Autodesk Inventor part; units mm, degrees
ref_plane "YZ Plane" through (0, 0, 0) normal (1, 0, 0) x (0, 1, 0)
ref_plane "XZ Plane" through (0, 0, 0) normal (0, 1, 0) x (-1, 0, 0)
ref_plane "XY Plane" through (0, 0, 0) normal (0, 0, 1) x (1, 0, 0)
sketch "Sketch1" plane through (0, 0, 0) normal (0, 0, 1) x (1, 0, 0)
  line L0 (-750, 67.5235) -> (750, 67.5235)
  line L1 (750, 67.5235) -> (750, 0)
  line L2 (750, 0) -> (-750, 0)
  line L3 (-750, 0) -> (-750, 67.5235)
  point P0 (0, 0)
  point P1 (0, 0)
  dimension "d0" = 1500
  dimension "d1" = 67.5235
extrude "Plate1" add sketch "Sketch1" along normal blind 2
sketch "Sketch2" plane through (750, 2, 0) normal (0, -1, 0) x (1, 0, 0)
  line L0 (-1500, 0) -> (0, 0)
  line L1 (0, 0) -> (0, 30)
  line L2 (0, 30) -> (-1500, 30)
  line L3 (-1500, 30) -> (-1500, 0)
edge flange "Flange1" height 30 angle 90 thickness 2 bend radius 2.75 thickness toward (0, -1, 0) relief round relief width 2 relief depth 1 edges at (0, 0, 2) wall of the first edge with corners at (-750, 2, 0) (750, 2, 0) (750, 2, 30) (-750, 2, 30)
bend "Bend1"
corner "Corner1"
sketch "Sketch5" plane through (0, 0, 0) normal (0, 0, -1) x (-1, 0, 0)
  line L0 (750, 67.5235) -> (-750, 67.5235)
  line L1 (-1, 30) -> (-1, 67.5235)
  line L2 (750, 0) -> (-750, 0)
  line L3 (-1, 30) -> (1, 30)
  line L4 (1, 30) -> (1, 67.5235)
  point P0 (0, 0)
  point P1 (0, 30)
  point P2 (0, 0)
  dimension "d27" = 2
  dimension "d28" = 30
extrude "Extrusion1" cut sketch "Sketch5" against normal through all
pattern_linear "Rectangular Pattern1" count 3 spacing 500 along (1, 0, 0) of "Extrusion1" first direction both ways yes
sketch "Sketch6" plane through (0, 0, 0) normal (0, 0, -1) x (-1, 0, 0)
  line L0 (-750, 67.5235) -> (-750, 4.75)
  circle A0 centre (-750, 67.5235) radius 22.5
  line L1 (-750, 67.5235) -> (750, 67.5235)
  line L2 (-1, 30) -> (-1, 67.5235)
  line L3 (-499, 67.5235) -> (-499, 30)
  line L4 (-1, 30) -> (-499, 30) construction
  circle A1 centre (-250, 67.5235) radius 22.5
  point P0 (0, 0)
  point P1 (-727.5, 67.5235)
  point P2 (-750, 45.0235)
  point P3 (-250, 30)
  dimension "d24" = 45
extrude "Extrusion2" cut sketch "Sketch6" along normal mid plane 30 contours L1 A0 L0 | A1 L1 | L1 A1 picked at (-748.3311, 52.7115)
mirror "Mirror1" about plane through (0, 0, 0) normal (1, 0, 0) of "Extrusion2"
sketch "Sketch7" plane through (0, 0, 2) normal (0, 0, 1) x (1, 0, 0)
  arc A0 (-750, 45.0235) -> (-727.5, 67.5235) centre (-750, 67.5235) ccw
  line L0 (-750, 4.75) -> (-750, 45.0235)
  line L1 (-750, 4.75) -> (750, 4.75)
  line L2 (750, 45.0235) -> (750, 4.75)
  arc A1 (727.5, 67.5235) -> (750, 45.0235) centre (750, 67.5235) ccw
  line L3 (501, 67.5235) -> (727.5, 67.5235)
  line L4 (501, 67.5235) -> (501, 30)
  line L5 (501, 30) -> (499, 30)
  line L6 (499, 30) -> (499, 67.5235)
  line L7 (1, 67.5235) -> (227.5, 67.5235)
  line L8 (1, 67.5235) -> (1, 30)
  line L9 (1, 30) -> (-1, 30)
  line L10 (-1, 30) -> (-1, 67.5235)
  line L11 (-499, 67.5235) -> (-272.5, 67.5235)
  line L12 (-499, 67.5235) -> (-499, 30)
  line L13 (-499, 30) -> (-501, 30)
  line L14 (-501, 30) -> (-501, 67.5235)
  line L15 (-727.5, 67.5235) -> (-501, 67.5235)
  line L16 (650, 4.75) -> (650, 67.5235) construction
  line L17 (-750, 4.75) -> (750, 4.75)
  circle A2 centre (650, 36.1368) radius 5
  line L18 (272.5, 67.5235) -> (499, 67.5235)
  arc A3 (227.5, 67.5235) -> (272.5, 67.5235) centre (250, 67.5235) ccw
  line L19 (-227.5, 67.5235) -> (-1, 67.5235)
  arc A4 (-272.5, 67.5235) -> (-227.5, 67.5235) centre (-250, 67.5235) ccw
  point P0 (0, 0)
  dimension "d29" = 100
  dimension "d30" = 10
extrude "Extrusion3" [suppressed]
mirror "Mirror2" [suppressed]
sketch "Sketch8" plane through (0, 0, 2) normal (0, 0, 1) x (1, 0, 0)
  line L0 (494, 62.5235) -> (494, 50.5235) construction
  line L1 (494, 50.5235) -> (294, 50.5235) construction
  line L2 (294, 50.5235) -> (294, 62.5235) construction
  line L3 (294, 62.5235) -> (494, 62.5235) construction
  line L4 (501, 67.5235) -> (727.5, 67.5235)
  line L5 (272.5, 67.5235) -> (499, 67.5235)
  point P0 (0, 0)
  dimension "d33" = 200
  dimension "d34" = 12
  dimension "d37" = 5
  dimension "d38" = 5
mark "Mark2"
equation "\"d1\" = Стрингер_3"
equation "\"d27\" = d18"
equation "\"d2\" = Thickness"
equation "\"d3\" = BendReliefWidth"
equation "\"d4\" = BendReliefDepth"
equation "\"d5\" = MinimumRemnant"
equation "\"d6\" = TransitionRadius"
equation "\"d9\" = BendRadius"
equation "\"d10\" = CornerReliefSize"
equation "\"d11\" = GapSize"
equation "\"d12\" = JacobiRadiusSize"
equation "\"BendReliefWidth\" = Thickness"
equation "\"BendReliefDepth\" = 0.5 * Thickness"
equation "\"CornerReliefSize\" = 4 * Thickness"
equation "\"MinimumRemnant\" = 2 * Thickness"
equation "\"TransitionRadius\" = BendRadius"
equation "\"JacobiRadiusSize\" = BendRadius"
equation "\"GapSize\" = Thickness"
equation "\"d18\" = Thickness"
properties part number "MSC 053 stringer board #" material "Stainless Steel"
Read the model definition and answer for the solid it produces. Units are mm, in the model's axes. A direction names the side the tool comes from. Round coordinates to 2 decimals unless told otherwise and drop trailing zeros. Order: outer loops, then holes, each group sorted by start corner. A loop starts at its lowest first (then second) coordinate and runs counter-clockwise, first axis right, second up.
1) The part is cut by section A-A on y = 55.5. Write down the section's boundary in (x, z).
2) Straight lines are drawn through the part: L1, parallel to Y at x = -579, z = 24.5; L2, parallel to Y at x = -668.5, z = 1.5. For each, find the intervals that lie inside material, in ascending order.
3) The part is cut by section B-B on x = -250. Write down the section's boundary in (y, z).
4) The part is cut by section D-D on x = -412. Write down the section's boundary in (y, z), plus the area to 3 significant figures.
5) The part is cut by section C-C on z = 17.25. Write down the section's boundary in (x, y), plus the area to 3 significant figures.
6) For faces 1 (the face through (-750, 15.7, 1.7)), 2 (the face through (-10, 37, 2)), determine the directions among +Z, -Z, +X, -X, +Y, -Y from which every point of the face is accessible in a straight line to the end or side of a thin tool.
7) Flat-ended cylindrical pins translate along their axes: pin 1 (2 mm diameter, centred on y = 49, z = 0.5, fed in from +X); pin 2 (2 mm diameter, centred on y = 52, z = 1, fed in from -X); pin 3 (3 mm diameter, centred on x = 503.5, y = 19.5, fed in from +Z); pin 4 (2 mm diameter, centred on x = -499.5, z = 1, fed in from +Y). Find the tip coordinate at first contact, or state that the pin passes through.
Resolved:
1. outline: (-730.98, 0) - (-501, 0) - (-501, 2) - (-730.98, 2) - close; (-499, 0) - (-269.02, 0) - (-269.02, 2) - (-499, 2) - close; (-230.98, 0) - (-1, 0) - (-1, 2) - (-230.98, 2) - close; (1, 0) - (230.98, 0) - (230.98, 2) - (1, 2) - close; (269.02, 0) - (499, 0) - (499, 2) - (269.02, 2) - close; (501, 0) - (730.98, 0) - (730.98, 2) - (501, 2) - close
2. L1: y = 0 to 2
2. L2: y = 1.29 to 67.52
3. outline: (0, 4.75) arc R4.75 ccw to (4.75, 0) - (45.02, 0) - (45.02, 2) - (4.75, 2) arc R2.75 cw to (2, 4.75) - (2, 30) - (0, 30) - close
4. outline: (0, 4.75) arc R4.75 ccw to (4.75, 0) - (67.52, 0) - (67.52, 2) - (4.75, 2) arc R2.75 cw to (2, 4.75) - (2, 30) - (0, 30) - close
4. area: 188 mm2
5. outline: (-750, 0) - (750, 0) - (750, 2) - (-750, 2) - close
5. area: 3,000 mm2
6. face 1: +Z, -Z, -X, +Y, -Y
6. face 2: +Z, +X, -X, +Y
7. pin 1: stops at x = 738.82
7. pin 2: stops at x = -734.73
7. pin 3: stops at z = 2
7. pin 4: stops at y = 67.52
